from build123d import *

# Parameters (mm, degrees)
F0_W     = 165
F0_H     = 75
F1_DEPTH = 3.048
F2_R     = 5.25
F3_DEPTH = 3.048
F4_R     = 10
F5_DEPTH = 3.048
F6_SIZE  = 3.175


# Not quite as in the source:
# - a pattern or mirror of a feature is missing from the dataset's text; its kind, count and spacing are read off the source's solid


with BuildPart() as f1:
    # F0 (on Front) → F1 (new body)
    with BuildSketch(Plane.XZ):
        with Locations((0, 37.5)):
            Rectangle(F0_W, F0_H)
    extrude(amount=F1_DEPTH)

    # F2 (on face) → F3 (cut)
    with BuildSketch(Plane.XZ.offset(3.048)):
        with Locations((-60.96, 17.5)):
            Circle(F2_R)
    f3 = extrude(amount=-F3_DEPTH, mode=Mode.SUBTRACT)

    # F3_copies: F3 across plane
    add(f3.mirror(Plane(origin=(0, 0, 0), x_dir=(0, 0, 1), z_dir=(1, 0, 0))), mode=Mode.SUBTRACT)

    # F4 (on face) → F5 (cut)
    with BuildSketch(Plane.XZ.offset(3.048)):
        with Locations((0, 58.5)):
            Circle(F4_R)
    extrude(amount=-F5_DEPTH, mode=Mode.SUBTRACT)

    # F6
    f6_edges = [f1.edges().sort_by_distance(p)[0] for p in [
        (-82.5, -1.524, 75),
        (-82.5, -1.524, 0),
        (82.5, -1.524, 0),
        (82.5, -1.524, 75),
    ]]
    chamfer(f6_edges, length=F6_SIZE)


solid = f1.part
Here's how the part is built. I have some questions about the finished solid (model axes, mm). Round coordinates to 2 decimals unless told otherwise and drop trailing zeros. Write each loop counter-clockwise with the first axis right and the second up, starting at its lowest first coordinate (ties: lowest second). Pieces come first, ordered by that corner, then holes.
1. Suppose I cut it at C-C (y = -2.35). List the corners of the cut face in (x, z) for me (3 decimals).
2. I need wall thicknesses on L1, parallel to Z at x = 60.96, y = -2.3; L2, parallel to Z at x = 0, y = -0.75; L3, parallel to X at y = -0.85, z = 66. Which ranges of each line are inside material? Lowest first, please.
3. If we mould it in two halves opening along Z, with no side actions, what happens to faces 1 (the cylindrical face through (-2.17, -1.55, 48.74)), 2 (the flat face through (-1, -2, 0)), 3 (the flat face through (-1, 0, 38))? For each: released by +Z, released by -Z, zero draft, split by the parting line, or undercut.
4. Suppose I cut it at A-A (x = 60.96). List the corners of the cut face in (y, z) for me, and give its area (3 significant figures).
5. Suppose I cut it at B-B (z = 66.5). List the corners of the cut face in (x, y) for me, and give its area (3 significant figures).
Answer sheet:
1. outline: (-82.5, 3.175) - (-79.325, 0) - (79.325, 0) - (82.5, 3.175) - (82.5, 71.825) - (79.325, 75) - (-79.325, 75) - (-82.5, 71.825) - close; hole circle Ø10.5 at (-60.96, 17.5); hole circle Ø20 at (0, 58.5); hole circle Ø10.5 at (60.96, 17.5)
2. L1: z = 0 to 12.25, 22.75 to 75
2. L2: z = 0 to 48.5, 68.5 to 75
2. L3: x = -82.5 to -6.61, 6.61 to 82.5
3. face 1: undercut
3. face 2: released by -Z
3. face 3: zero draft
4. outline: (-3.05, 0) - (0, 0) - (0, 12.25) - (-3.05, 12.25) - close; (-3.05, 22.75) - (0, 22.75) - (0, 75) - (-3.05, 75) - close
4. area: 197 mm2
5. outline: (-82.5, -3.05) - (-6, -3.05) - (-6, 0) - (-82.5, 0) - close; (6, -3.05) - (82.5, -3.05) - (82.5, 0) - (6, 0) - close
5. area: 466 mm2
